```python
from build123d import *

# Parameters (mm, degrees)
BOSS_EXTRUDE2_DEPTH = 50
SKETCH2_R           = 2.5
CUT_EXTRUDE1_DEPTH  = 347
SKETCH3_R           = 2.5
CUT_EXTRUDE2_DEPTH  = 288.757501625


with BuildPart() as part:
    # Sketch1 → Boss-Extrude2 (new body)
    with BuildSketch(Plane.XY):
        Polygon((0, 0), (-85.5, -234), (-85.5, -287.757501625), (-78.5, -287.757501625), (-78.5, -235.238794474), (4.894944135, -7), (170.105055865, -7), (253.5, -235.238794474), (253.5, -287.757501625), (260.5, -287.757501625), (260.5, -234), (175, 0), align=None)
    extrude(amount=BOSS_EXTRUDE2_DEPTH)

    # Sketch2 → Cut-Extrude1 (cut, through all)
    with BuildSketch(Plane(origin=(260.5, 0, 0), x_dir=(0, 0, -1), z_dir=(1, 0, 0))):
        with Locations((-25, -275.891246781)):
            Circle(SKETCH2_R)
    extrude(amount=-CUT_EXTRUDE1_DEPTH, mode=Mode.SUBTRACT)

    # Sketch3 → Cut-Extrude2 (cut, through all)
    with BuildSketch(Plane(origin=(0, 0, 0), x_dir=(1, 0, 0), z_dir=(0, 1, 0))):
        with Locations((112.5, -25)):
            Circle(SKETCH3_R)
        with Locations((62.5, -25)):
            Circle(SKETCH3_R)
    extrude(amount=-CUT_EXTRUDE2_DEPTH, mode=Mode.SUBTRACT)


solid = part.part
```
Check sheet for the modelled part. Datum: model origin and axes. Units: mm. A direction names the side the tool comes from. Round coordinates to 2 decimals unless told otherwise and drop trailing zeros. Write each loop counter-clockwise with the first axis right and the second up, starting at its lowest first coordinate (ties: lowest second). Pieces come first, ordered by that corner, then holes. Notation, with made-up numbers: M 38.5,34 L 77.5,34 A20 ccw 77.5,46 Z; hole C -9.5,11 d11. An arc over 180 degrees is marked long. Write item = value, one per line. Start each with the question number.
1. Section check C-C, the plane x = 22.5. Record the cut outline in (y, z), then the cut area to 3 significant figures.
2. Section check B-B, the plane z = 35. Record the cut outline in (x, y).
3. Scan lines: line 1 (Z direction, x = 112.5, y = -5); line 2 (X direction, y = -274, z = 40); line 3 (Y direction, x = 57.5, z = 37). Record each from-to range of solid material in increasing order. Write a range as [from, to].
4. Section check A-A, the plane y = -144. Record the cut outline in (x, z).
5. Release check for a two-part mould opening along X. For faces 1 (the flat face through (-85.5, -261, 25)), 2 (the flat face through (-78.5, -262, 25)), 3 (the flat face through (-16, -58, 0)) record: pulls with the +X half, pulls with the -X half, needs draft (parallel to the pull), parting line crosses it, or undercut.
6. Section check D-D, the plane x = -50.5. Record the cut outline in (y, z), then the cut area to 3 significant figures.
7. Gauge pin test, flat ends, axial feed: pin 1 (1.5 mm diameter, centred on x = 52.5, z = 37, fed in from -Y); pin 2 (8 mm diameter, centred on y = -116.5, z = 6, fed in from +X); pin 3 (4 mm diameter, centred on x = 62.5, z = 25, fed in from +Y); pin 4 (10 mm diameter, centred on y = -126, z = 28, fed in from -X). Record the tip position at first contact, or that the pin passes through.
8. Tool access check on faces 4 (the flat face through (260.5, -261, 25)), 5 (the flat face through (86, -7, 25)). Record the directions out of +Z, -Z, +X, -X, +Y, -Y that give a thin tool (end or side, any length) a straight path to the whole face; none if there is none.
Results found:
q1.outline = M -7,0 L 0,0 L 0,50 L -7,50 Z
q1.area = 350 mm^2
q2.outline = M -85.5,-287.76 L -78.5,-287.76 L -78.5,-235.24 L 4.89,-7 L 170.11,-7 L 253.5,-235.24 L 253.5,-287.76 L 260.5,-287.76 L 260.5,-234 L 175,0 L 0,0 L -85.5,-234 Z
q3.line_1 = [0, 22.5], [27.5, 50]
q3.line_2 = [-85.5, -78.5], [253.5, 260.5]
q3.line_3 = [-7, 0]
q4.outline = M -52.62,0 L -45.16,0 L -45.16,50 L -52.62,50 Z; M 220.16,0 L 227.62,0 L 227.62,50 L 220.16,50 Z
q5.face_1 = pulls with the -X half
q5.face_2 = undercut
q5.face_3 = needs draft
q6.outline = M -158.61,0 L -138.21,0 L -138.21,50 L -158.61,50 Z
q6.area = 1,020 mm^2
q7.pin_1 = -7
q7.pin_2 = 219.03
q7.pin_3 = through
q7.pin_4 = -47.87
q8.face_4 = +Z, -Z, +X, +Y, -Y
q8.face_5 = +Z, -Z, -Y
